Could you check a few things on this model? Use its own coordinates, in mm. Round coordinates to 2 decimals unless told otherwise and drop trailing zeros. Loops run counter-clockwise (first coordinate to the right, second up) from the corner with the lowest first, then second, coordinate; pieces in that order, holes last. Notation, with made-up numbers: M 43,-20 L 85,-20 A23 cw 85,8 Z; hole C 51,6.5 d5. An arc over 180 degrees is marked long. One line per item, written item: value. Start each with the question number.
Q1. I'm going to push flat-ended pins straight in: pin 1 Ø4 at (x, z) = (604, 7.5) entering from -Y; pin 2 Ø7 at (x, y) = (130, -16.04) entering from +Z; pin 3 Ø3.5 at (x, y) = (670, -16.04) entering from -Z; pin 4 Ø1 at (x, y) = (911, -24) entering from +Z. Where does each tip first touch, or does it pass through?
Q2. Imagine slicing it at A-A (x = 808). Please give me the cut outline in (y, z), then the cut area to 3 significant figures.
Q3. Please list where these lines run through material, in increasing order: line 1 along Y through (x, z) = (670, 4); line 2 along Y through (x, z) = (550, 8); line 3 along Y through (x, z) = (1077.5, 17.25).
from build123d import *

# Parameters (mm, degrees)
F1_DEPTH = 1170
F2_R     = 3
F3_DEPTH = 18
F4_R     = 5
F5_DEPTH = 7


with BuildPart() as f1:
    # F0 (on Right) → F1 (new body)
    with BuildSketch(Plane.YZ):
        with BuildLine():
            Line((-26.041336, 5), (-26.041336, 0))
            Line((-26.041336, 0), (-6.041336, 0))
            Line((-6.041336, 0), (-6.041336, 5))
            ThreePointArc((-6.041336, 5), (-9.041336, 8), (-6.041336, 11))
            Line((-6.041336, 11), (-6.041336, 15))
            ThreePointArc((-6.041336, 15), (-8.162657, 15.87868), (-9.041336, 18))
            Line((-9.041336, 18), (-23.041336, 18))
            ThreePointArc((-23.041336, 18), (-23.920016, 15.87868), (-26.041336, 15))
            Line((-26.041336, 15), (-26.041336, 11))
            ThreePointArc((-26.041336, 11), (-23.041336, 8), (-26.041336, 5))
        make_face()
    extrude(amount=F1_DEPTH)

    # F2 (on face) → F3 (cut)
    with BuildSketch(Plane.XY.offset(18)):
        with Locations((10, -16.041336)):
            Circle(F2_R)
        with Locations((70, -16.041336)):
            Circle(F2_R)
        with Locations((130, -16.041336)):
            Circle(F2_R)
        with Locations((190, -16.041336)):
            Circle(F2_R)
        with Locations((250, -16.041336)):
            Circle(F2_R)
        with Locations((310, -16.041336)):
            Circle(F2_R)
        with Locations((370, -16.041336)):
            Circle(F2_R)
        with Locations((430, -16.041336)):
            Circle(F2_R)
        with Locations((490, -16.041336)):
            Circle(F2_R)
        with Locations((550, -16.041336)):
            Circle(F2_R)
        with Locations((610, -16.041336)):
            Circle(F2_R)
        with Locations((670, -16.041336)):
            Circle(F2_R)
        with Locations((730, -16.041336)):
            Circle(F2_R)
        with Locations((790, -16.041336)):
            Circle(F2_R)
        with Locations((850, -16.041336)):
            Circle(F2_R)
        with Locations((910, -16.041336)):
            Circle(F2_R)
        with Locations((970, -16.041336)):
            Circle(F2_R)
        with Locations((1030, -16.041336)):
            Circle(F2_R)
        with Locations((1090, -16.041336)):
            Circle(F2_R)
        with Locations((1150, -16.041336)):
            Circle(F2_R)
        with Locations((1210, -16.041336)):
            Circle(F2_R)
        with Locations((1270, -16.041336)):
            Circle(F2_R)
        with Locations((1330, -16.041336)):
            Circle(F2_R)
        with Locations((1390, -16.041336)):
            Circle(F2_R)
        with Locations((1450, -16.041336)):
            Circle(F2_R)
        with Locations((1510, -16.041336)):
            Circle(F2_R)
        with Locations((1570, -16.041336)):
            Circle(F2_R)
        with Locations((1630, -16.041336)):
            Circle(F2_R)
        with Locations((1690, -16.041336)):
            Circle(F2_R)
        with Locations((1750, -16.041336)):
            Circle(F2_R)
        with Locations((1810, -16.041336)):
            Circle(F2_R)
        with Locations((1870, -16.041336)):
            Circle(F2_R)
        with Locations((1930, -16.041336)):
            Circle(F2_R)
        with Locations((1990, -16.041336)):
            Circle(F2_R)
    extrude(amount=-F3_DEPTH, mode=Mode.SUBTRACT)

    # F4 (on face) → F5 (cut)
    with BuildSketch(Plane.XY.offset(18)):
        with Locations((10, -16.041336)):
            Circle(F4_R)
        with Locations((70, -16.041336)):
            Circle(F4_R)
        with Locations((130, -16.041336)):
            Circle(F4_R)
        with Locations((190, -16.041336)):
            Circle(F4_R)
        with Locations((250, -16.041336)):
            Circle(F4_R)
        with Locations((310, -16.041336)):
            Circle(F4_R)
        with Locations((370, -16.041336)):
            Circle(F4_R)
        with Locations((430, -16.041336)):
            Circle(F4_R)
        with Locations((490, -16.041336)):
            Circle(F4_R)
        with Locations((550, -16.041336)):
            Circle(F4_R)
        with Locations((610, -16.041336)):
            Circle(F4_R)
        with Locations((670, -16.041336)):
            Circle(F4_R)
        with Locations((730, -16.041336)):
            Circle(F4_R)
        with Locations((790, -16.041336)):
            Circle(F4_R)
        with Locations((850, -16.041336)):
            Circle(F4_R)
        with Locations((910, -16.041336)):
            Circle(F4_R)
        with Locations((970, -16.041336)):
            Circle(F4_R)
        with Locations((1030, -16.041336)):
            Circle(F4_R)
        with Locations((1090, -16.041336)):
            Circle(F4_R)
    extrude(amount=-F5_DEPTH, mode=Mode.SUBTRACT)


solid = f1.part
Report:
1. pin 1: stops at y = -24.38
1. pin 2: stops at z = 11
1. pin 3: passes through
1. pin 4: stops at z = 16.41
2. outline: M -26.04,0 L -6.04,0 L -6.04,5 A3 cw -6.04,11 L -6.04,15 A3 cw -9.04,18 L -23.04,18 A3 cw -26.04,15 L -26.04,11 A3 cw -26.04,5 Z
2. area: 318 mm²
3. line 1: y = -26.04 to -19.04, -13.04 to -6.04
3. line 2: y = -23.04 to -19.04, -13.04 to -9.04
3. line 3: y = -23.14 to -8.95
